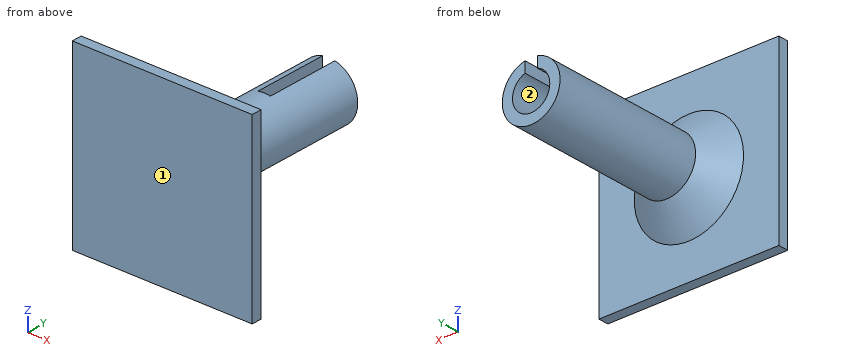
from build123d import *

# Parameters (mm, degrees)
SKETCH2_R           = 11.25
SKETCH2_R_2         = 7.25
BOSS_EXTRUDE1_DEPTH = 71
BOSS_EXTRUDE2_START = -4
SKETCH2_6_W         = 70
SKETCH2_6_H         = 70
SKETCH2_6_R         = 11.25
SKETCH2_6_R_2       = 7.25
BOSS_EXTRUDE2_DEPTH = 4
CHAMFER1_SIZE       = 10
SKETCH6_W           = 4.8
SKETCH6_H           = 29.123834
CUT_EXTRUDE2_DEPTH  = 25


with BuildPart() as part:
    # Sketch2 → Boss-Extrude1 (new body)
    with BuildSketch(Plane(origin=(0, 0, 0), x_dir=(1, 0, 0), z_dir=(0, 1, 0))):
        with Locations(Location((0, 0, 0), (0, 0, 270))):
            Circle(SKETCH2_R)
        with Locations(Location((0, 0, 0), (0, 0, 270))):
            Circle(SKETCH2_R_2, mode=Mode.SUBTRACT)
    extrude(amount=BOSS_EXTRUDE1_DEPTH)

    # Sketch2_6 → Boss-Extrude2 (add)
    # profile 1 of 3: a face of its own
    with BuildSketch(Plane(origin=(0, 0, 0), x_dir=(1, 0, 0), z_dir=(0, 1, 0)).offset(BOSS_EXTRUDE2_START)):
        Rectangle(SKETCH2_6_W, SKETCH2_6_H)
        with Locations(Location((0, 0, 0), (0, 0, 270))):
            Circle(SKETCH2_6_R, mode=Mode.SUBTRACT)
    # profile 2 of 3: a face of its own
    with BuildSketch(Plane(origin=(0, 0, 0), x_dir=(1, 0, 0), z_dir=(0, 1, 0)).offset(BOSS_EXTRUDE2_START)):
        with Locations(Location((0, 0, 0), (0, 0, 270))):
            Circle(SKETCH2_6_R)
        with Locations(Location((0, 0, 0), (0, 0, 270))):
            Circle(SKETCH2_6_R_2, mode=Mode.SUBTRACT)
    # profile 3 of 3: a face of its own
    with BuildSketch(Plane(origin=(0, 0, 0), x_dir=(1, 0, 0), z_dir=(0, 1, 0)).offset(BOSS_EXTRUDE2_START)):
        with Locations(Location((0, 0, 0), (0, 0, 270))):
            Circle(SKETCH2_6_R_2)
    extrude(amount=BOSS_EXTRUDE2_DEPTH)

    # Chamfer1
    chamfer1_edges = [part.edges().sort_by_distance(p)[0] for p in [
        (0, 0, -11.25),
    ]]
    chamfer(chamfer1_edges, length=CHAMFER1_SIZE)

    # Sketch6 → Cut-Extrude2 (cut)
    with BuildSketch(Plane.XY):
        with Locations((0, 56.438083)):
            Rectangle(SKETCH6_W, SKETCH6_H)
    extrude(amount=CUT_EXTRUDE2_DEPTH, mode=Mode.SUBTRACT)


solid = part.part
Source: CAD feature listing. Evaluate the final solid. Frame: model axes, mm. Face numbers are marked on the shaded views. A direction names the side the tool comes from. Coordinates: 2 decimals unless noted, no trailing zeros. Loops run counter-clockwise (first coordinate to the right, second up) from the corner with the lowest first, then second, coordinate; pieces in that order, holes last. Notation, with made-up numbers: (40, 7.5) - (57, 7.5) arc R10 ccw to (57, 24.5) - close; hole circle Ø7 at (69.25, 64.5). An arc over 180 degrees is marked (long way). One line per question, with ' | ' between items.
1) Section C-C, the plane y = 17. Return loops of the section in (x, z).
Report:
outline: circle Ø22.5 at (0, 0); hole circle Ø14.5 at (0, 0)
2) First-contact query: P1, Ø1, axis at x = 5.5, z = 14.5, coming from the +Y side; P2, Ø6, axis at x = 9, y = 58.5, coming from the +Z side; P3, Ø2, axis at y = 57.5, z = 9.5, coming from the +X side. Flat tips, straight axial feed; report the tip coordinate or a pass-through.
Report:
P1: stops at y = 6.24 | P2: stops at z = 9.52 | P3: stops at x = 7.37
3) Section A-A, the plane x = 0. Return loops of the section in (y, z), then the cut area to 3 significant figures.
Report:
outline: (-4, -35) - (0, -35) - (0, -21.25) - (10, -11.25) - (71, -11.25) - (71, -7.25) - (0, -7.25) - (0, 7.25) - (41.88, 7.25) - (41.88, 11.25) - (10, 11.25) - (0, 21.25) - (0, 35) - (-4, 35) - close | area: 832 mm²
4) Line query: line 1 along X through (y, z) = (53, 0); line 2 along Y through (x, z) = (-1, 4); line 3 along Z through (x, y) = (-4, 44). Output: solid intervals per line, ascending.
Report:
line 1: x = -11.25 to -7.25, 7.25 to 11.25 | line 2: y = -4 to 0 | line 3: z = -10.51 to -6.05, 6.05 to 10.51
5) Set-up query: the marked faces 1 and 2. Return all of +Z, -Z, +X, -X, +Y, -Y with unobstructed straight access to the full face (end or side cutting, diameter ignored); none if empty.
Report:
face 1: +Z, -Z, +X, -X, -Y | face 2: +Y
6) Section B-B, the plane z = 0. Return loops of the section in (x, y), then the cut area to 3 significant figures.
Report:
outline: (-35, -4) - (35, -4) - (35, 0) - (21.25, 0) - (11.25, 10) - (11.25, 71) - (7.25, 71) - (7.25, 0) - (-7.25, 0) - (-7.25, 71) - (-11.25, 71) - (-11.25, 10) - (-21.25, 0) - (-35, 0) - close | area: 948 mm²
7) Section D-D, the plane y = 52. Return loops of the section in (x, z).
Report:
outline: (-2.4, 6.84) - (-2.4, 10.99) arc R11.25 ccw (long way) to (2.4, 10.99) - (2.4, 6.84) arc R7.25 cw (long way) to start
